from build123d import *

# Parameters (mm, degrees)
SKETCH1_W           = 1676.4
SKETCH1_H           = 1676.4
BOSS_EXTRUDE1_DEPTH = 10
SKETCH1_2_W         = 1696.4
SKETCH1_2_H         = 1696.4
SKETCH1_2_W_2       = 1676.4
SKETCH1_2_H_2       = 1676.4
EXTRUDE_THIN1_DEPTH = 533.4


with BuildPart() as part:
    # Sketch1 → Boss-Extrude1 (new body)
    with BuildSketch(Plane(origin=(0, 0, 0), x_dir=(1, 0, 0), z_dir=(0, 1, 0))):
        Rectangle(SKETCH1_W, SKETCH1_H)
    extrude(amount=BOSS_EXTRUDE1_DEPTH)

    # Sketch1<2> → Extrude-Thin1 (add)
    with BuildSketch(Plane(origin=(0, 0, 0), x_dir=(1, 0, 0), z_dir=(0, 1, 0))):
        Rectangle(SKETCH1_2_W, SKETCH1_2_H)
        Rectangle(SKETCH1_2_W_2, SKETCH1_2_H_2, mode=Mode.SUBTRACT)
    extrude(amount=EXTRUDE_THIN1_DEPTH)


solid = part.part
Design review of the part built by this model. Coordinates are the model's own, in mm. A direction names the side the tool comes from. Coordinates: 2 decimals unless noted, no trailing zeros. Loops run counter-clockwise (first coordinate to the right, second up) from the corner with the lowest first, then second, coordinate; pieces in that order, holes last. Notation, with made-up numbers: (70.5, -28.5) -> (113.5, -28.5) arc R12 ccw to (113.5, -13.5) -> close; hole circle Ø2 at (-26.75, 30.5). An arc over 180 degrees is marked (long way). Use a Markdown table: item, result. Add a question column.
Item 1: Machinability: for faces 1 (the flat face through (-12, 263, -848.2)), 2 (the flat face through (-838.2, 268, 12)), which of the approach directions +Z, -Z, +X, -X, +Y, -Y give a long, thin tool a straight path to every point of the face, cutting with its end or side? Answer none if there is none.
Item 2: Clearance check with flat-ended pins moving along their axes: P1, Ø1.5, axis at x = -6.5, z = -563.5, coming from the +Y side; P2, Ø10, axis at x = 582.5, z = 479.5, coming from the -Y side. State where each tip first meets the part, or that it passes through.
Item 3: Wall thickness on L1, parallel to X at y = 38, z = -289; L2, parallel to Y at x = -578, z = -551.5: over which ranges is each line inside the solid? List them lowest first. Write a range as from..to.
Item 4: The part is to be moulded in two halves that separate along X. For faces 3 (the flat face through (-12, 263, 848.2)), 4 (the flat face through (-848.2, 263, 12)), 5 (the flat face through (-12, 268, -838.2)), say which applies: +X half, -X half, draft (parallel to the pull), parting line (faces both ways), or undercut.
Item 5: We need section B-B, the plane x = -491.5. Write out the cut boundary in (y, z).
Item 6: We need section A-A, the plane y = 312. Write out the cut boundary in (x, z).
Item 7: We need section C-C, the plane z = -626. Write out the cut boundary in (x, y), and give its area (3 significant figures).
Numbers:
| question | item | result |
|---|---|---|
| 1 | face 1 | -Z, +X, -X, +Y, -Y |
| 1 | face 2 | +Y |
| 2 | P1 | stops at y = 10 |
| 2 | P2 | stops at y = 0 |
| 3 | L1 | x = -848.2..-838.2, 838.2..848.2 |
| 3 | L2 | y = 0..10 |
| 4 | face 3 | draft |
| 4 | face 4 | -X half |
| 4 | face 5 | undercut |
| 5 | outline | (0, -848.2) -> (533.4, -848.2) -> (533.4, -838.2) -> (10, -838.2) -> (10, 838.2) -> (533.4, 838.2) -> (533.4, 848.2) -> (0, 848.2) -> close |
| 6 | outline | (-848.2, -848.2) -> (848.2, -848.2) -> (848.2, 848.2) -> (-848.2, 848.2) -> close; hole (-838.2, -838.2) -> (838.2, -838.2) -> (838.2, 838.2) -> (-838.2, 838.2) -> close |
| 7 | outline | (-848.2, 0) -> (848.2, 0) -> (848.2, 533.4) -> (838.2, 533.4) -> (838.2, 10) -> (-838.2, 10) -> (-838.2, 533.4) -> (-848.2, 533.4) -> close |
| 7 | area | 27,400 mm^2 |
